Here's how the part is built. I have some questions about the finished solid (model axes, mm). Face numbers are marked on the shaded views. A direction names the side the tool comes from. Round coordinates to 2 decimals unless told otherwise and drop trailing zeros. Order: outer loops, then holes, each group sorted by start corner. A loop starts at its lowest first (then second) coordinate and runs counter-clockwise, first axis right, second up. Notation, with made-up numbers: (-2, 8.5) -> (51, 8.5) arc R13 cw to (51, 23.5) -> close; hole circle Ø9 at (-4.75, -9.75). An arc over 180 degrees is marked (long way). Use a Markdown table: item, result. Add a question column.
(1) On a 3-axis mill with a long thin cutter (end or side, diameter ignored), from which of +Z, -Z, +X, -X, +Y, -Y can I reach the whole of each face in a straight line? I mean the marked faces 5 and 6. Say none if no direction works.
(2) Thinking about a two-plate mould opening in X: for the marked faces 1, 2, 3 and 4, which applies, pulls with the +X half, pulls with the -X half, needs draft (parallel to the pull), parting line crosses it, or undercut?
(3) I'm going to push flat-ended pins straight in: P1, Ø5, axis at x = 86.5, y = 36.5, coming from the -Z side; P2, Ø1.5, axis at y = 72, z = -26, coming from the +X side; P3, Ø10, axis at y = 22.5, z = -20.5, coming from the -X side. Where does each tip first touch, or does it pass through?
(4) I want a section at B-B, the plane y = 64.5. Please give me the cut outline in (x, z).
(5) I want a section at C-C, the plane x = 123. Please give me the cut outline in (y, z).
(6) If I drill on probe 1 along X at (y, z) = (25.5, -24); probe 2 along Z at (x, y) = (84.5, 44.5); probe 3 along Z at (x, y) = (59.5, 19), over which ranges is the centre line in solid material (lowest first)?
(7) I want a section at A-A, the plane z = -19.5. Please give me the cut outline in (x, y).
(8) I want a section at D-D, the plane z = -6.5. Please give me the cut outline in (x, y), then the cut area to 3 significant figures.
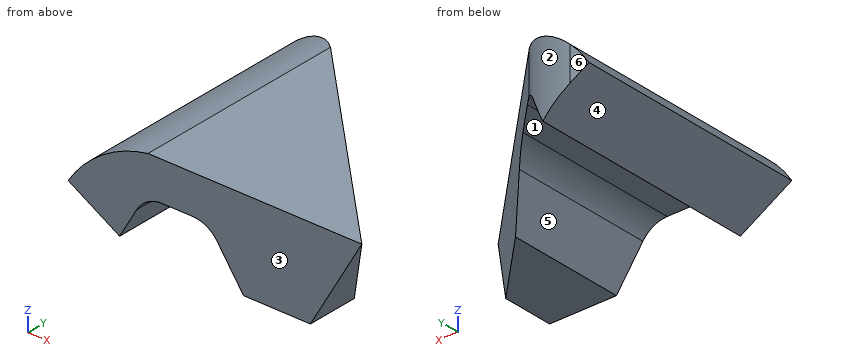
from build123d import *

# Parameters (mm, degrees)
BOSS_EXTRUDE1_DEPTH = 80
CUT_EXTRUDE1_DEPTH  = 60
FILLET1_R           = 30
FILLET3_R           = 10


with BuildPart() as part:
    # Sketch31 → Boss-Extrude1 (new body)
    with BuildSketch(Plane(origin=(0, 0, 0), x_dir=(1, 0, 0), z_dir=(0, 1, 0))):
        with BuildLine():
            Line((78, 0), (150, 0))
            Line((150, 0), (132.679491924, 30))
            Line((132.679491924, 30), (110.179491924, 30))
            Line((110.179491924, 30), (98.275963775, 13))
            Line((98.275963775, 13), (82.859757015, 13))
            ThreePointArc((82.859757015, 13), (77.860100275, 14.33954779), (74.199899362, 17.999313504))
            Line((74.199899362, 17.999313504), (68.440162758, 27.973643859))
            Line((68.440162758, 27.973643859), (51.120447452, 17.972270867))
            ThreePointArc((51.120447452, 17.972270867), (62.6510159, 6.130700387), (78, 0))
        make_face()
    extrude(amount=BOSS_EXTRUDE1_DEPTH)

    # Sketch32 → Cut-Extrude1 (cut)
    with BuildSketch(Plane.XY):
        Polygon((70, 80), (150, 0), (150, 80), align=None)
    extrude(amount=-CUT_EXTRUDE1_DEPTH, mode=Mode.SUBTRACT)

    # Fillet1
    fillet1_edges = [part.edges().sort_by_distance(p)[0] for p in [
        (70, 80, -13.766443848),
    ]]
    fillet(fillet1_edges, radius=FILLET1_R)

    # Fillet3
    fillet3_edges = [part.edges().sort_by_distance(p)[0] for p in [
        (98.275963775, 25.862018113, -13),
    ]]
    fillet(fillet3_edges, radius=FILLET3_R)


solid = part.part
Taken from the geometry:
| question | item | result |
|---|---|---|
| 1 | face 5 | -Z, +Y, -Y |
| 1 | face 6 | +Z, -Z, +X, -X, +Y |
| 2 | face 1 | undercut |
| 2 | face 2 | pulls with the +X half |
| 2 | face 3 | needs draft |
| 2 | face 4 | pulls with the -X half |
| 3 | P1 | stops at z = -13 |
| 3 | P2 | stops at x = 70.01 |
| 3 | P3 | stops at x = 51.12 |
| 4 | outline | (51.12, -17.97) -> (68.44, -27.97) -> (74.2, -18) arc R10 cw to (82.86, -13) -> (85.5, -13) -> (85.5, 0) -> (78, 0) arc R39.76 ccw to start |
| 5 | outline | (0, -30) -> (27, -30) -> (27, 0) -> (0, 0) -> close |
| 6 | probe 1 | x = 61.56 to 70.73, 105.98 to 124.5 |
| 6 | probe 2 | z = -13 to 0 |
| 6 | probe 3 | z = -22.81 to -8.47 |
| 7 | outline | (53.77, 0) -> (73.33, 0) -> (73.33, 75.53) arc R30 ccw to (57.57, 80) -> (53.77, 80) -> close; (102.83, 0) -> (138.74, 0) -> (138.74, 11.26) -> (102.83, 47.17) -> close |
| 8 | outline | (62.11, 0) -> (146.25, 0) -> (146.25, 3.75) -> (78.79, 71.21) arc R30 ccw to (62.11, 79.66) -> close |
| 8 | area | 3,810 mm2 |
